Geometry: final body of the model. Coordinates: model frame, mm. A direction names the side the tool comes from. Coordinates: 2 decimals unless noted, no trailing zeros. Loops run counter-clockwise (first coordinate to the right, second up) from the corner with the lowest first, then second, coordinate; pieces in that order, holes last. Notation, with made-up numbers: (32, 88.25) -> (55, 88.25) arc R12 cw to (55, 104.25) -> close; hole circle Ø6 at (-39, 67). An arc over 180 degrees is marked (long way). One line per item, written item: value. Start each with the question number.
Item 1: Set-up query: faces 1 (the flat face through (2, -6, 5)), 2 (the cylindrical face through (0.35, -16.43, 6.44)), 3 (the cylindrical face through (18.26, -17.67, 0.62)), 4 (the flat face through (18, -10, 10)). Return all of +Z, -Z, +X, -X, +Y, -Y with unobstructed straight access to the full face (end or side cutting, diameter ignored); none if empty.
Item 2: Contact query for flat-ended pins moving along their axis: pin 1 Ø1 at (x, z) = (11.5, -5) entering from +Y; pin 2 Ø4 at (x, z) = (-8, 0) entering from -Y; pin 3 Ø2.5 at (x, z) = (8, 0) entering from +Y. Output: stop coordinate, or through.
Item 3: Ray query, probe 1 along Z at (x, y) = (0, -17); probe 2 along Y at (x, z) = (18, -1.25); probe 3 along X at (y, z) = (-9, 7.25). Return the intervals inside material, ascending. Write a range as from..to.
Item 4: Mould query, pull axis Z, two halves, no side actions, for faces 5 (the flat face through (0, -12, 12.5)), 6 (the cylindrical face through (-6.4, -16.43, 0.07)), 7 (the cylindrical face through (-28.092, -15.899, 11.268)). Classes: +Z half, -Z half, draft (parallel to the pull), parting line (faces both ways), or undercut.
Item 5: Section query A-A on x = 18. Return loops of the section in (y, z).
Item 6: Section query B-B on y = -16.5. Give the number of separate pieces and of enclosed holes in the cut face, then the cut area to 3 significant figures.
from build123d import *

# Parameters (mm, degrees)
F0_W           = 65
F0_H           = 21
F0_R           = 5.1
F1_DEPTH       = 25
F3_D           = 2.4
F3_CBORE_D     = 4
F3_CBORE_DEPTH = 2.5
F4_SIZE        = 0.49999
F5_R           = 5.1
F6_DEPTH       = 3.5
F8_D           = 3.2
F8_DEPTH       = 8
F8_TIP         = 0.9613769904
F10_D          = 3.2
F10_DEPTH      = 10
F10_TIP        = 0.9613769904
F11_R          = 5.1
F12_DEPTH      = 6


# Not quite as in the source:
# - a fillet or chamfer is up to 0.001 mm smaller than in the source, because OpenCascade refuses the exact size


with BuildPart() as f1:
    # F0 (on Front) → F1 (new body)
    with BuildSketch(Plane.XZ):
        with Locations((0, 2)):
            Rectangle(F0_W, F0_H)
        Circle(F0_R, mode=Mode.SUBTRACT)
    extrude(amount=F1_DEPTH)

    # F3 (through all)
    with Locations(Plane.XY.offset(12.5)):
        with Locations((-30, -8.5), (-30, -16.5), (-18, -8.5), (-18, -16.5), (18, -16.5), (18, -8.5), (30, -8.5), (30, -16.5)):
            CounterBoreHole(F3_D / 2, F3_CBORE_D / 2, F3_CBORE_DEPTH)

    # F4 (size 0.5 in the source; OpenCascade refuses exactly that, so slightly less here)
    f4_edges = [f1.edges().sort_by_distance(p)[0] for p in [
        (-32.5, -12.5, 12.5),
        (32.5, -12.5, 12.5),
    ]]
    chamfer(f4_edges, length=F4_SIZE)

    # F5 (on face) → F6 (cut)
    with BuildSketch(Plane.XZ.offset(25)):
        with BuildLine():
            ThreePointArc((6.9821200219, -8.5), (9.9449313784, -4.7008871375), (11, 0))
            ThreePointArc((11, 0), (-4.7008871375, 9.9449313784), (-6.9821200219, -8.5))
            Line((-6.9821200219, -8.5), (6.9821200219, -8.5))
        make_face()
        Circle(F5_R, mode=Mode.SUBTRACT)
    extrude(amount=-F6_DEPTH, mode=Mode.SUBTRACT)

    # F8
    with Locations(Plane.XY.offset(12.5)):
        with Locations((12.5, -6.25), (12.5, -18.75), (-12.5, -6.25), (-12.5, -18.75)):
            Hole(F8_D / 2, depth=F8_DEPTH)
            with Locations((0, 0, -(F8_DEPTH + F8_TIP / 2))):  # 118° drill point
                Cone(0, F8_D / 2, F8_TIP, mode=Mode.SUBTRACT)

    # F10
    with Locations(Plane.XZ.offset(21.5)):
        with Locations((-8, 0), (0, 8), (8, 0)):
            Hole(F10_D / 2, depth=F10_DEPTH)
            with Locations((0, 0, -(F10_DEPTH + F10_TIP / 2))):  # 118° drill point
                Cone(0, F10_D / 2, F10_TIP, mode=Mode.SUBTRACT)

    # F11 (on face) → F12 (cut)
    with BuildSketch(Plane(origin=(0, 0, 0), x_dir=(-1, 0, 0), z_dir=(0, 1, 0))):
        with BuildLine():
            ThreePointArc((4.2426406871, -8.5), (8.0794519161, -4.9972449146), (9.5, 0))
            ThreePointArc((9.5, 0), (-4.9972449146, 8.0794519161), (-4.2426406871, -8.5))
            Line((-4.2426406871, -8.5), (4.2426406871, -8.5))
        make_face()
        Circle(F11_R, mode=Mode.SUBTRACT)
        Circle(F11_R)
    extrude(amount=-F12_DEPTH, mode=Mode.SUBTRACT)


solid = f1.part
Reply:
1. face 1: +Y
1. face 2: -Y
1. face 3: +Z, -Z
1. face 4: +Z
2. pin 1: stops at y = 0
2. pin 2: stops at y = -21.5
2. pin 3: stops at y = -6
3. probe 1: z = -8.5..-5.1, 5.1..6.4, 9.6..12.5
3. probe 2: y = -25..-17.7, -15.3..-9.7, -7.3..0
3. probe 3: x = -32.5..-31.09, -28.91..-19.09, -16.91..16.91, 19.09..28.91, 31.09..32.5
4. face 5: +Z half
4. face 6: undercut
4. face 7: draft
5. outline: (-25, -8.5) -> (-17.7, -8.5) -> (-17.7, 10) -> (-18.5, 10) -> (-18.5, 12.5) -> (-25, 12.5) -> close; (-15.3, -8.5) -> (-9.7, -8.5) -> (-9.7, 10) -> (-10.5, 10) -> (-10.5, 12.5) -> (-14.5, 12.5) -> (-14.5, 10) -> (-15.3, 10) -> close; (-7.3, -8.5) -> (0, -8.5) -> (0, 12.5) -> (-6.5, 12.5) -> (-6.5, 10) -> (-7.3, 10) -> close
6. separate pieces: 5
6. enclosed holes: 4
6. area: 1,040 mm²
